For this review, take the finished solid that the model builds, in its own axes (mm). A direction names the side the tool comes from. Give positions to 0.01 mm unless a question says otherwise; leave off trailing zeros. Loops run counter-clockwise (first coordinate to the right, second up) from the corner with the lowest first, then second, coordinate; pieces in that order, holes last. Notation, with made-up numbers: M -38,58 L -17,58 A19 ccw -17,94 Z; hole C -36,53 d7. An arc over 180 degrees is marked long. Use CSV: the item, a comma, the result in double quotes. Start each with the question number.
1. Insertion check: P1, Ø2, axis at x = -17, y = 2.5, coming from the -Z side; P2, Ø1, axis at y = 2.5, z = 15, coming from the -X side; P3, Ø6.5, axis at x = -35, z = 0, coming from the +Y side; P4, Ø4.5, axis at x = 0, z = -35, coming from the +Y side. Each pin has a flat end and moves straight along its axis. Give the tip position at first contact, or say it passes through.
2. The part is to be moulded in two halves that separate along Z. For faces 1 (the face through (9, 0, 1)), 2 (the face through (32.56, 1.97, -0.54)), 3 (the face through (-17.235, 1.972, 41.569)), say which applies: pulls with the +Z half, pulls with the -Z half, needs draft (parallel to the pull), parting line crosses it, or undercut.
3. Tool access review of faces 4 (the face through (11, 4, 9)), 5 (the face through (0, 7, -11)), 6 (the face through (6, 13, 0)): name each direction out of +Z, -Z, +X, -X, +Y, -Y from which nothing blocks a thin tool from reaching the whole face with its end or side.
4. Take a section at A-A, the plane z = 0. Write out the cut boundary in (x, y).
5. Take a section at D-D, the plane z = 35. Write out the cut boundary in (x, y).
6. Take a section at C-C, the plane y = 2.25. Write out the cut boundary in (x, z), and give its area (3 significant figures).
7. To check wall thickness, follow line 1 (X direction, y = 3, z = 0); line 2 (X direction, y = 2.25, z = 9); line 3 (Y direction, x = -11, z = -18). State the ranges of each line that lie inside material, in increasing order. Write a range as [from, to].
8. Take a section at B-B, the plane x = 0. Write out the cut boundary in (y, z), and give its area (3 significant figures).
from build123d import *

# Parameters (mm, degrees)
SKETCH1_R           = 45
SKETCH1_R_2         = 14
SKETCH1_R_3         = 2.5
BOSS_EXTRUDE1_DEPTH = 4
SKETCH1_3_R         = 14
BOSS_EXTRUDE2_DEPTH = 13
CUT_EXTRUDE1_DEPTH  = 65.953829756


with BuildPart() as part:
    # Sketch1 → Boss-Extrude1 (new body)
    # profile 1 of 2: a face of its own
    with BuildSketch(Plane(origin=(0, 0, 0), x_dir=(1, 0, 0), z_dir=(0, 1, 0))):
        with Locations(Location((0, 0, 0), (0, 0, 270))):
            Circle(SKETCH1_R)
        Circle(SKETCH1_R_2, mode=Mode.SUBTRACT)
        with Locations(Location((-35, 0, 0), (0, 0, 270))):
            Circle(SKETCH1_R_3, mode=Mode.SUBTRACT)
        with Locations(Location((0, -35, 0), (0, 0, 270))):
            Circle(SKETCH1_R_3, mode=Mode.SUBTRACT)
        with Locations(Location((35, 0, 0), (0, 0, 270))):
            Circle(SKETCH1_R_3, mode=Mode.SUBTRACT)
        with Locations(Location((0, 35, 0), (0, 0, 270))):
            Circle(SKETCH1_R_3, mode=Mode.SUBTRACT)
    # profile 2 of 2: a face of its own
    with BuildSketch(Plane(origin=(0, 0, 0), x_dir=(1, 0, 0), z_dir=(0, 1, 0))):
        Circle(SKETCH1_R_2)
    extrude(amount=BOSS_EXTRUDE1_DEPTH)

    # Sketch1_3 → Boss-Extrude2 (add)
    with BuildSketch(Plane(origin=(0, 0, 0), x_dir=(1, 0, 0), z_dir=(0, 1, 0))):
        with Locations(Location((0, 0, 0), (0, 0, 90))):
            Circle(SKETCH1_3_R)
    extrude(amount=BOSS_EXTRUDE2_DEPTH)

    # Sketch3 → Cut-Extrude1 (cut, through all)
    with BuildSketch(Plane(origin=(0, 13, 0), x_dir=(1, 0, 0), z_dir=(0, 1, 0))):
        with BuildLine():
            Line((-5, -6), (-5, 6))
            ThreePointArc((-5, 6), (0, 11), (5, 6))
            Line((5, 6), (5, -6))
            ThreePointArc((5, -6), (0, -11), (-5, -6))
        make_face()
    extrude(amount=-CUT_EXTRUDE1_DEPTH, mode=Mode.SUBTRACT)


solid = part.part
Result set:
1,P1,"z = -42.06"
1,P2,"x = -42.6"
1,P3,"y = 4"
1,P4,"through"
2,face 1,"needs draft"
2,face 2,"undercut"
2,face 3,"parting line crosses it"
3,face 4,"+Y"
3,face 5,"+Y, -Y"
3,face 6,"+Z, -Z, +X, -X, +Y"
4,outline,"M -45,0 L -37.5,0 L -37.5,4 L -45,4 Z; M -32.5,0 L -5,0 L -5,13 L -14,13 L -14,4 L -32.5,4 Z; M 5,0 L 32.5,0 L 32.5,4 L 14,4 L 14,13 L 5,13 Z; M 37.5,0 L 45,0 L 45,4 L 37.5,4 Z"
5,outline,"M -28.28,0 L -2.5,0 L -2.5,4 L -28.28,4 Z; M 2.5,0 L 28.28,0 L 28.28,4 L 2.5,4 Z"
6,outline,"C 0,0 d90; hole C -35,0 d5; hole M -5,-6 A5 ccw 5,-6 L 5,6 A5 ccw -5,6 Z; hole C 0,-35 d5; hole C 0,35 d5; hole C 35,0 d5"
6,area,"6,080 mm2"
7,line 1,"[-45, -37.5], [-32.5, -5], [5, 32.5], [37.5, 45]"
7,line 2,"[-44.09, -4], [4, 44.09]"
7,line 3,"[0, 4]"
8,outline,"M 0,-45 L 4,-45 L 4,-37.5 L 0,-37.5 Z; M 0,-32.5 L 4,-32.5 L 4,-14 L 13,-14 L 13,-11 L 0,-11 Z; M 0,11 L 13,11 L 13,14 L 4,14 L 4,32.5 L 0,32.5 Z; M 0,37.5 L 4,37.5 L 4,45 L 0,45 Z"
8,area,"286 mm2"
